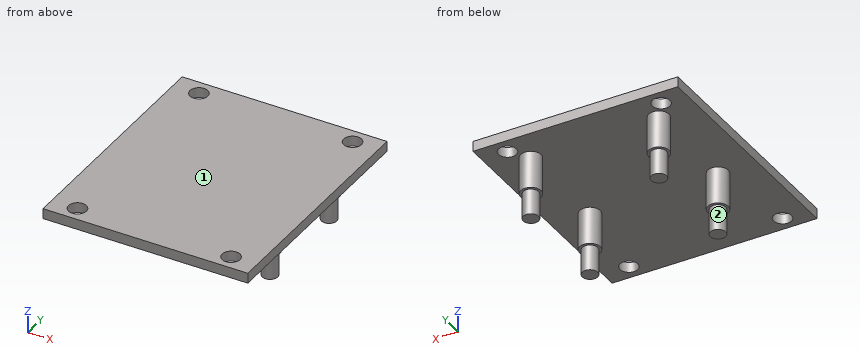
Autodesk Inventor part; units mm, degrees
ref_plane "YZ Plane" through (0, 0, 0) normal (1, 0, 0) x (0, 1, 0)
ref_plane "XZ Plane" through (0, 0, 0) normal (0, 1, 0) x (-1, 0, 0)
ref_plane "XY Plane" through (0, 0, 0) normal (0, 0, 1) x (1, 0, 0)
sketch "Sketch1" plane through (0, 0, 0) normal (0, 0, 1) x (1, 0, 0)
  line L0 (0, 0) -> (40, 0)
  line L1 (40, 0) -> (40, 51)
  line L2 (40, 51) -> (0, 51)
  line L3 (0, 51) -> (0, 0)
  circle A0 centre (5, 3) radius 1.75
  circle A1 centre (12.5, 3) radius 1.75
  circle A2 centre (20, 3) radius 1.75
  circle A3 centre (27.5, 3) radius 1.75
  circle A4 centre (35, 3) radius 1.75
  line L4 (7.5, 20.5) -> (32.5, 20.5)
  line L5 (32.5, 20.5) -> (32.5, 40.5)
  line L6 (32.5, 40.5) -> (7.5, 40.5)
  line L7 (7.5, 40.5) -> (7.5, 20.5)
  line L8 (7.5, 20.5) -> (32.5, 40.5) construction
  line L9 (32.5, 20.5) -> (7.5, 40.5) construction
  circle A5 centre (32.5, 40.5) radius 2
  circle A6 centre (32.5, 20.5) radius 2
  circle A7 centre (7.5, 20.5) radius 2
  circle A8 centre (7.5, 40.5) radius 2
  circle A9 centre (35, 44.1) radius 1.75
  line L10 (0, 47.1) -> (40, 47.1)
  line L11 (40, 47.1) -> (40, 51)
  line L12 (40, 51) -> (0, 51)
  line L13 (0, 51) -> (0, 47.1)
  circle A10 centre (5, 44.1) radius 1.75
  point P0 (20, 51)
  point P1 (20, 30.5)
  point P2 (40, 25.5)
  point P3 (40, 47.1)
  dimension "d0" = 3.5
  dimension "d3" = 7.5
  dimension "d8" = 40
  dimension "d10" = 4
  dimension "d11" = 4
  dimension "d12" = 4
  dimension "d13" = 4
  dimension "d14" = 20
  dimension "d15" = 25
  dimension "d16" = 5
  dimension "d21" = 3
  dimension "d22" = 41.1
  dimension "d23" = 3
  dimension "d25" = 27.5
extrude "Extrusion1" add sketch "Sketch1" along normal blind 2 contours L3 L10 L1 L0 | A1 | A2 | A3 | L7 A7 L4 | L4 A7 L7 | A7 L7 A8 L6 A5 L5 A6 L4 | A6 L5 L4 | L4 L5 A6 | A8 L6 L7 | L7 L6 A8 | A5 L6 L5 | L5 L6 A5
extrude "Extrusion2" add sketch "Sketch1" against normal blind 7.3 contours L7 A7 L4 | L4 A7 L7 | A6 L5 L4 | L4 L5 A6 | A8 L6 L7 | L7 L6 A8 | A5 L6 L5 | L5 L6 A5
sketch "Sketch2" plane through (32.5, 20.5, -7.3) normal (0, 0, -1) x (-1, 0, 0)
  circle A0 centre (0, 20) radius 2
  circle A1 centre (0, 0) radius 2
  circle A2 centre (25, 20) radius 2
  circle A3 centre (25, 0) radius 2
  circle A4 centre (0, 20) radius 1.5
  circle A5 centre (0, 0) radius 1.5
  circle A6 centre (25, 0) radius 1.5
  circle A7 centre (25, 20) radius 1.5
  point P0 (32.5, -20.5)
  dimension "d26" = 3
  dimension "d27" = 3
  dimension "d28" = 3
  dimension "d29" = 3
extrude "Extrusion3" add sketch "Sketch2" along normal blind 5 contours A4 | A5 | A6 | A7
properties part number "HOLDER_MARKER_ROBOTAT" material "ABS Plastic"
The model under review builds one solid part; all positions refer to its coordinate system, in mm. Face numbers are marked on the shaded views. Coordinates: 2 decimals unless noted, no trailing zeros. Write each loop counter-clockwise with the first axis right and the second up, starting at its lowest first coordinate (ties: lowest second). Pieces come first, ordered by that corner, then holes.
1) The part is to be moulded in two halves that separate along Y. For the marked faces 1 and 2, say which applies: pulls with the +Y half, pulls with the -Y half, needs draft (parallel to the pull), parting line crosses it, or undercut.
2) We need section D-D on x = 22. State the section outline as (y, z) points.
3) We need section B-B on y = 40.5. State the section outline as (x, z) points, then the cut area to 3 significant figures.
4) We need section A-A on y = 3. State the section outline as (x, z) points.
5) To check wall thickness, follow probe 1 along Y at (x, z) = (35, 0.75); probe 2 along Z at (x, y) = (17.5, 7); probe 3 along X at (y, z) = (19.5, -8). State the ranges of each line that lie inside material, in increasing order.
6) We need section C-C on z = -8.75. State the section outline as (x, y) points, then the cut area to 3 significant figures.
7) Clearance check with flat-ended pins moving along their axes: pin 1 Ø6 at (y, z) = (26, -10.5) entering from +X; pin 2 Ø1.5 at (x, z) = (7.5, -8) entering from -Y; pin 3 Ø20 at (x, y) = (21.5, 34.5) entering from -Z. State where each tip first meets the part, or that it passes through.
Answer list:
1. face 1: needs draft
1. face 2: undercut
2. outline: (0, 0) - (47.1, 0) - (47.1, 2) - (0, 2) - close
3. outline: (0, 0) - (5.5, 0) - (5.5, -7.3) - (6, -7.3) - (6, -12.3) - (9, -12.3) - (9, -7.3) - (9.5, -7.3) - (9.5, 0) - (30.5, 0) - (30.5, -7.3) - (31, -7.3) - (31, -12.3) - (34, -12.3) - (34, -7.3) - (34.5, -7.3) - (34.5, 0) - (40, 0) - (40, 2) - (0, 2) - close
3. area: 168 mm2
4. outline: (0, 0) - (3.25, 0) - (3.25, 2) - (0, 2) - close; (6.75, 0) - (33.25, 0) - (33.25, 2) - (6.75, 2) - close; (36.75, 0) - (40, 0) - (40, 2) - (36.75, 2) - close
5. probe 1: y = 0 to 1.25, 4.75 to 42.35, 45.85 to 47.1
5. probe 2: z = 0 to 2
5. probe 3: x = 6.38 to 8.62, 31.38 to 33.62
6. outline: circle Ø3 at (7.5, 20.5); circle Ø3 at (7.5, 40.5); circle Ø3 at (32.5, 20.5); circle Ø3 at (32.5, 40.5)
6. area: 28.3 mm2
7. pin 1: passes through
7. pin 2: stops at y = 18.5
7. pin 3: stops at z = 0
